Design review of the part built by this model. Coordinates are the model's own, in mm. A direction names the side the tool comes from. Round coordinates to 2 decimals unless told otherwise and drop trailing zeros. Write each loop counter-clockwise with the first axis right and the second up, starting at its lowest first coordinate (ties: lowest second). Pieces come first, ordered by that corner, then holes.
from build123d import *
from OCP.BRepAlgoAPI import BRepAlgoAPI_Cut
from OCP.TopTools import TopTools_ListOfShape

# Parameters (mm, degrees)
SKETCH2_W           = 124.17
SKETCH2_H           = 119.38
BOSS_EXTRUDE1_DEPTH = 3.18
SKETCH3_R           = 1.905
SKETCH3_R_2         = 11.685
CUT_EXTRUDE1_DEPTH  = 23.18
SKETCH5_W           = 1.59
SKETCH5_H           = 120
CUT_EXTRUDE2_DEPTH  = 10
SKETCH6_R           = 1.905
CUT_EXTRUDE3_DEPTH  = 5


with BuildPart() as part:
    # Sketch2 → Boss-Extrude1 (new body)
    with BuildSketch(Plane(origin=(0, -1.061487407, 0), x_dir=(1, 0, 0), z_dir=(0, 0, 1))):
        with Locations((0.708693295, -25.828343308)):
            Rectangle(SKETCH2_W, SKETCH2_H)
    extrude(amount=BOSS_EXTRUDE1_DEPTH)

    # Sketch3 → Cut-Extrude1 (cut)
    with BuildSketch(Plane.XY):
        with Locations((-42.776306705, 27.348169285)):
            Circle(SKETCH3_R)
        with Locations((41.729693295, 17.090169285)):
            Circle(SKETCH3_R_2)
        with Locations((-42.776306705, -81.127830715)):
            Circle(SKETCH3_R)
        with Locations((57.343693295, -13.339830715)):
            Circle(SKETCH3_R)
        with Locations((57.343693295, -40.439830715)):
            Circle(SKETCH3_R)
    extrude(amount=CUT_EXTRUDE1_DEPTH, mode=Mode.SUBTRACT)


with BuildPart() as cut_extrude2_tool:
    # Sketch5 → Cut-Extrude2 (new body)
    with BuildSketch(Plane.ZY.offset(61.376306705)):
        with Locations((0.794999799, -27.199831736)):
            Rectangle(SKETCH5_W, SKETCH5_H)
    extrude(amount=-CUT_EXTRUDE2_DEPTH)


with BuildPart() as part_1:
    add(part.part)

    # Cut-Extrude2: cut by cut_extrude2_tool, with a tolerance
    cut_extrude2_stock = TopTools_ListOfShape()
    cut_extrude2_stock.Append(part_1.part.wrapped)
    cut_extrude2_tools = TopTools_ListOfShape()
    cut_extrude2_tools.Append(cut_extrude2_tool.part.wrapped)
    cut_extrude2_cut = BRepAlgoAPI_Cut()
    cut_extrude2_cut.SetArguments(cut_extrude2_stock)
    cut_extrude2_cut.SetTools(cut_extrude2_tools)
    cut_extrude2_cut.SetFuzzyValue(0.00001)
    cut_extrude2_cut.Build()
    add(Compound.cast(cut_extrude2_cut.Shape()).solids(), mode=Mode.REPLACE)

    # Sketch6 → Cut-Extrude3 (cut)
    with BuildSketch(Plane(origin=(0, 0, 1.589999799), x_dir=(-1, 0, 0), z_dir=(0, 0, -1))):
        with Locations(Location((56.376306705, 14.720168264, 0), (0, 0, 90))):
            Circle(SKETCH6_R)
        with Locations(Location((56.376306705, -21.449831736, 0), (0, 0, 90))):
            Circle(SKETCH6_R)
        with Locations(Location((56.376306705, -72.579830715, 0), (0, 0, 90))):
            Circle(SKETCH6_R)
        with Locations(Location((56.376306705, -3.369831736, 0), (0, 0, 90))):
            Circle(SKETCH6_R)
    extrude(amount=-CUT_EXTRUDE3_DEPTH, mode=Mode.SUBTRACT)


solid = part_1.part
1) The part is to be moulded in two halves that separate along X. For faces 3 (the face through (62.794, -28, 2)), 4 (the face through (-57.54, -22.96, 2.37)), 5 (the face through (5, -26, 0)), say which applies: pulls with the +X half, pulls with the -X half, needs draft (parallel to the pull), parting line crosses it, or undercut.
2) Add section C-C on y = -58. State the section outline as (x, z) points, and give its area (3 significant figures).
3) Add section A-A on y = -3.5. State the section outline as (x, z) points, and give its area (3 significant figures).
4) Add section B-B on z = 2.5. Count the separate pieces of the cut face and the enclosed holes in it, and give its area (3 significant figures).
5) For line 1 along Y through (x, z) = (42.5, 1.3); line 2 along X through (y, z) = (-33.5, 0.3); line 3 along X through (y, z) = (-71, 1.8), list the stretches that pass through material, from the lowest coordinate up.
6) For faces 1 (the face through (-56, -28, 1.59)), 2 (the face through (-40.959, -80.556, 1.568)), list the 3-axis set-ups (+Z, -Z, +X, -X, +Y, -Y) from which the entire face can be reached by the end or side of a thin tool; tool diameter is ignored.
7) For P1, Ø4.5, axis at x = -56.38, y = -72.58, coming from the -Z side; P2, Ø1.3, axis at y = -41, z = 0.5, coming from the -X side; P3, Ø6, axis at x = -42.78, y = -81.13, coming from the -Z side, all flat-tipped, find the tip position at first contact; note any pin that passes through.
8) Add section D-D on y = 10.5. State the section outline as (x, z) points, and give its area (3 significant figures).
Computed:
1. face 3: pulls with the +X half
1. face 4: undercut
1. face 5: needs draft
2. outline: (-61.38, 1.59) - (-51.38, 1.59) - (-51.38, 0) - (62.79, 0) - (62.79, 3.18) - (-61.38, 3.18) - close
2. area: 379 mm2
3. outline: (-61.38, 1.59) - (-58.28, 1.59) - (-58.28, 3.18) - (-61.38, 3.18) - close; (-54.48, 1.59) - (-51.38, 1.59) - (-51.38, 0) - (62.79, 0) - (62.79, 3.18) - (-54.48, 3.18) - close
3. area: 373 mm2
4. separate pieces: 1
4. enclosed holes: 9
4. area: 14,300 mm2
5. line 1: y = -86.58 to 5.43, 28.75 to 32.8
5. line 2: x = -51.38 to 62.79
5. line 3: x = -61.38 to -57.44, -55.31 to 62.79
6. face 1: -Z, -X, +Y, -Y
6. face 2: +Z, -Z
7. P1: stops at z = 1.59
7. P2: stops at x = -51.38
7. P3: stops at z = 0
8. outline: (-61.38, 1.59) - (-51.38, 1.59) - (-51.38, 0) - (32.08, 0) - (32.08, 3.18) - (-61.38, 3.18) - close; (51.38, 0) - (62.79, 0) - (62.79, 3.18) - (51.38, 3.18) - close
8. area: 318 mm2
